from build123d import *

# Parameters (mm, degrees)
SKETCH_12_W         = 240
SKETCH_12_H         = 52
EXTRUDE_1_DEPTH     = 10
CUT_EXTRUDE_4_REACH = 125.191
SKETCH_11_R         = 1.5


with BuildPart() as part:
    # 草图12 → 凸台-拉伸1 (new body)
    with BuildSketch(Plane(origin=(0, 0, 0), x_dir=(1, 0, 0), z_dir=(0, 1, 0))):
        Rectangle(SKETCH_12_W, SKETCH_12_H)
    extrude(amount=EXTRUDE_1_DEPTH)

    # 草图11 → 切除-拉伸4 (cut, up to next)
    with BuildSketch(Plane(origin=(0, 0, 0), x_dir=(1, 0, 0), z_dir=(0, 1, 0)), mode=Mode.PRIVATE) as cut_extrude_4_sk1:
        with Locations(Location((-109.5, 15.5, 0), (0, 0, 270))):
            Circle(SKETCH_11_R)
    cut_extrude_4_tool1 = extrude(cut_extrude_4_sk1.sketch, amount=CUT_EXTRUDE_4_REACH, mode=Mode.PRIVATE) & part.part
    # 草图11 → 切除-拉伸4 (cut, up to next)
    with BuildSketch(Plane(origin=(0, 0, 0), x_dir=(1, 0, 0), z_dir=(0, 1, 0)), mode=Mode.PRIVATE) as cut_extrude_4_sk2:
        with Locations(Location((-78.5, 15.5, 0), (0, 0, 270))):
            Circle(SKETCH_11_R)
    cut_extrude_4_tool2 = extrude(cut_extrude_4_sk2.sketch, amount=CUT_EXTRUDE_4_REACH, mode=Mode.PRIVATE) & part.part
    # 草图11 → 切除-拉伸4 (cut, up to next)
    with BuildSketch(Plane(origin=(0, 0, 0), x_dir=(1, 0, 0), z_dir=(0, 1, 0)), mode=Mode.PRIVATE) as cut_extrude_4_sk3:
        with Locations(Location((-109.5, -15.5, 0), (0, 0, 270))):
            Circle(SKETCH_11_R)
    cut_extrude_4_tool3 = extrude(cut_extrude_4_sk3.sketch, amount=CUT_EXTRUDE_4_REACH, mode=Mode.PRIVATE) & part.part
    # 草图11 → 切除-拉伸4 (cut, up to next)
    with BuildSketch(Plane(origin=(0, 0, 0), x_dir=(1, 0, 0), z_dir=(0, 1, 0)), mode=Mode.PRIVATE) as cut_extrude_4_sk4:
        with Locations(Location((-78.5, -15.5, 0), (0, 0, 270))):
            Circle(SKETCH_11_R)
    cut_extrude_4_tool4 = extrude(cut_extrude_4_sk4.sketch, amount=CUT_EXTRUDE_4_REACH, mode=Mode.PRIVATE) & part.part
    # 草图11 → 切除-拉伸4 (cut, up to next)
    with BuildSketch(Plane(origin=(0, 0, 0), x_dir=(1, 0, 0), z_dir=(0, 1, 0)), mode=Mode.PRIVATE) as cut_extrude_4_sk5:
        with Locations(Location((78.5, 15.5, 0), (0, 0, 270))):
            Circle(SKETCH_11_R)
    cut_extrude_4_tool5 = extrude(cut_extrude_4_sk5.sketch, amount=CUT_EXTRUDE_4_REACH, mode=Mode.PRIVATE) & part.part
    # 草图11 → 切除-拉伸4 (cut, up to next)
    with BuildSketch(Plane(origin=(0, 0, 0), x_dir=(1, 0, 0), z_dir=(0, 1, 0)), mode=Mode.PRIVATE) as cut_extrude_4_sk6:
        with Locations(Location((109.5, 15.5, 0), (0, 0, 270))):
            Circle(SKETCH_11_R)
    cut_extrude_4_tool6 = extrude(cut_extrude_4_sk6.sketch, amount=CUT_EXTRUDE_4_REACH, mode=Mode.PRIVATE) & part.part
    # 草图11 → 切除-拉伸4 (cut, up to next)
    with BuildSketch(Plane(origin=(0, 0, 0), x_dir=(1, 0, 0), z_dir=(0, 1, 0)), mode=Mode.PRIVATE) as cut_extrude_4_sk7:
        with Locations(Location((109.5, -15.5, 0), (0, 0, 270))):
            Circle(SKETCH_11_R)
    cut_extrude_4_tool7 = extrude(cut_extrude_4_sk7.sketch, amount=CUT_EXTRUDE_4_REACH, mode=Mode.PRIVATE) & part.part
    # 草图11 → 切除-拉伸4 (cut, up to next)
    with BuildSketch(Plane(origin=(0, 0, 0), x_dir=(1, 0, 0), z_dir=(0, 1, 0)), mode=Mode.PRIVATE) as cut_extrude_4_sk8:
        with Locations(Location((78.5, -15.5, 0), (0, 0, 270))):
            Circle(SKETCH_11_R)
    cut_extrude_4_tool8 = extrude(cut_extrude_4_sk8.sketch, amount=CUT_EXTRUDE_4_REACH, mode=Mode.PRIVATE) & part.part
    # 草图11 → 切除-拉伸4 (cut, up to next)
    with BuildSketch(Plane(origin=(0, 0, 0), x_dir=(1, 0, 0), z_dir=(0, 1, 0)), mode=Mode.PRIVATE) as cut_extrude_4_sk9:
        with BuildLine():
            Line((-65, 17.05), (65, 17.05))
            ThreePointArc((65, 17.05), (66.55, 15.5), (65, 13.95))
            Line((65, 13.95), (-65, 13.95))
            ThreePointArc((-65, 13.95), (-66.55, 15.5), (-65, 17.05))
        make_face()
    cut_extrude_4_tool9 = extrude(cut_extrude_4_sk9.sketch, amount=CUT_EXTRUDE_4_REACH, mode=Mode.PRIVATE) & part.part
    # 草图11 → 切除-拉伸4 (cut, up to next)
    with BuildSketch(Plane(origin=(0, 0, 0), x_dir=(1, 0, 0), z_dir=(0, 1, 0)), mode=Mode.PRIVATE) as cut_extrude_4_sk10:
        with BuildLine():
            Line((-65, -13.95), (65, -13.95))
            ThreePointArc((65, -13.95), (66.55, -15.5), (65, -17.05))
            Line((65, -17.05), (-65, -17.05))
            ThreePointArc((-65, -17.05), (-66.55, -15.5), (-65, -13.95))
        make_face()
    cut_extrude_4_tool10 = extrude(cut_extrude_4_sk10.sketch, amount=CUT_EXTRUDE_4_REACH, mode=Mode.PRIVATE) & part.part
    add(cut_extrude_4_tool1.solids().sort_by_distance((-109.5, 0, -15.5))[0], mode=Mode.SUBTRACT)
    add(cut_extrude_4_tool2.solids().sort_by_distance((-78.5, 0, -15.5))[0], mode=Mode.SUBTRACT)
    add(cut_extrude_4_tool3.solids().sort_by_distance((-109.5, 0, 15.5))[0], mode=Mode.SUBTRACT)
    add(cut_extrude_4_tool4.solids().sort_by_distance((-78.5, 0, 15.5))[0], mode=Mode.SUBTRACT)
    add(cut_extrude_4_tool5.solids().sort_by_distance((78.5, 0, -15.5))[0], mode=Mode.SUBTRACT)
    add(cut_extrude_4_tool6.solids().sort_by_distance((109.5, 0, -15.5))[0], mode=Mode.SUBTRACT)
    add(cut_extrude_4_tool7.solids().sort_by_distance((109.5, 0, 15.5))[0], mode=Mode.SUBTRACT)
    add(cut_extrude_4_tool8.solids().sort_by_distance((78.5, 0, 15.5))[0], mode=Mode.SUBTRACT)
    add(cut_extrude_4_tool9.solids().sort_by_distance((0, 0, -15.5))[0], mode=Mode.SUBTRACT)
    add(cut_extrude_4_tool10.solids().sort_by_distance((0, 0, 15.5))[0], mode=Mode.SUBTRACT)


solid = part.part
Verification items for the finished model (mm, model axes). A direction names the side the tool comes from. Round coordinates to 2 decimals unless told otherwise and drop trailing zeros. Order: outer loops, then holes, each group sorted by start corner. A loop starts at its lowest first (then second) coordinate and runs counter-clockwise, first axis right, second up.
1. Section check B-B on y = 1.5. State how many separate pieces and enclosed holes the cut face has, then the cut area to 3 significant figures.
Final values:
separate pieces: 1
enclosed holes: 10
area: 11,600 mm2
2. Thickness scan on L1, parallel to Z at x = -78.5, y = 3.75; L2, parallel to X at y = 2, z = 15.5. Record the ranges inside material, lowest first.
Final values:
L1: z = -26 to -17, -14 to 14, 17 to 26
L2: x = -120 to -111, -108 to -80, -77 to -66.55, 66.55 to 77, 80 to 108, 111 to 120
3. Section check A-A on x = -35.5. Record the cut outline in (y, z).
Final values:
outline: (0, -26) - (10, -26) - (10, -17.05) - (0, -17.05) - close; (0, -13.95) - (10, -13.95) - (10, 13.95) - (0, 13.95) - close; (0, 17.05) - (10, 17.05) - (10, 26) - (0, 26) - close
4. Access from +Z, -Z, +X, -X, +Y, -Y to the whole of each face (thin tool, end or side, straight path). Record for faces 4 (the flat face through (-2, 0, 0)), 5 (the flat face through (1, 5, 17.05)).
Final values:
face 4: +Z, -Z, +X, -X, -Y
face 5: +Y, -Y
5. Release check for a two-part mould opening along X. For faces 1 (the flat face through (120, 5, 0)), 2 (the flat face through (-1, 5, 13.95)), 3 (the flat face through (-120, 5, 0)) record: +X half, -X half, draft (parallel to the pull), parting line (faces both ways), or undercut.
Final values:
face 1: +X half
face 2: undercut
face 3: -X half
